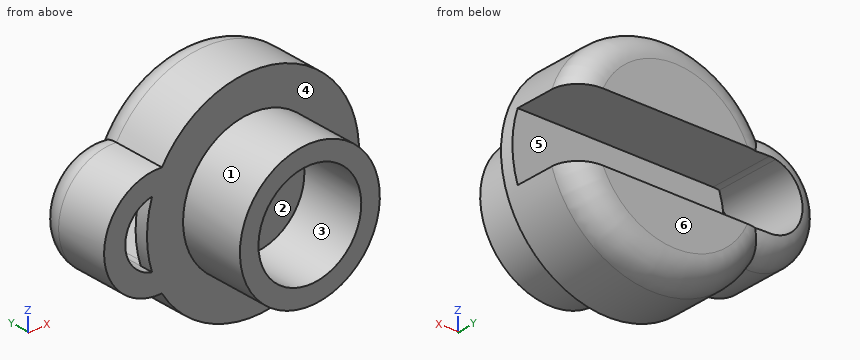
```python
from build123d import *

# Parameters (mm, degrees)
SKETCH1_R           = 3.3528
SKETCH1_R_2         = 2.4638
BOSS_EXTRUDE1_DEPTH = 3.175
SKETCH2_R           = 5.08
BOSS_EXTRUDE2_DEPTH = 3.81
BOSS_EXTRUDE3_START = -3.81
SKETCH3_R           = 5.08
SKETCH3_R_2         = 2.6035
SKETCH3_R_3         = 1.5875
BOSS_EXTRUDE3_DEPTH = 3.81
CUT_EXTRUDE1_START  = -3.175
CUT_EXTRUDE1_DEPTH  = 3.175
FILLET1_R           = 1.27


with BuildPart() as part:
    # Sketch1 → Boss-Extrude1 (new body)
    with BuildSketch(Plane(origin=(0, 0, 0), x_dir=(1, 0, 0), z_dir=(0, 1, 0))):
        with Locations(Location((0, 0, 0), (0, 0, 270))):
            Circle(SKETCH1_R)
        with Locations(Location((0, 0, 0), (0, 0, 270))):
            Circle(SKETCH1_R_2, mode=Mode.SUBTRACT)
    extrude(amount=BOSS_EXTRUDE1_DEPTH)

    # Sketch2 → Boss-Extrude2 (add)
    with BuildSketch(Plane(origin=(0, 3.175, 0), x_dir=(1, 0, 0), z_dir=(0, 1, 0))):
        with Locations(Location((0, 0, 0), (0, 0, 90))):
            Circle(SKETCH2_R)
    extrude(amount=BOSS_EXTRUDE2_DEPTH)

    # Sketch3 → Boss-Extrude3 (add)
    # profile 1 of 3: a face of its own
    with BuildSketch(Plane(origin=(0, 6.985, 0), x_dir=(1, 0, 0), z_dir=(0, 1, 0)).offset(BOSS_EXTRUDE3_START)):
        Circle(SKETCH3_R)
    # profile 2 of 3: a face of its own
    with BuildSketch(Plane(origin=(0, 6.985, 0), x_dir=(1, 0, 0), z_dir=(0, 1, 0)).offset(BOSS_EXTRUDE3_START)):
        with Locations((-4.533681302, 0)):
            Circle(SKETCH3_R_2)
        with Locations((-4.533681302, 0)):
            Circle(SKETCH3_R_3, mode=Mode.SUBTRACT)
    # profile 3 of 3: a face of its own
    with BuildSketch(Plane(origin=(0, 6.985, 0), x_dir=(1, 0, 0), z_dir=(0, 1, 0)).offset(BOSS_EXTRUDE3_START)):
        Circle(SKETCH3_R)
    extrude(amount=BOSS_EXTRUDE3_DEPTH)

    # Sketch4 → Cut-Extrude1 (cut)
    with BuildSketch(Plane(origin=(0, 6.985, 0), x_dir=(1, 0, 0), z_dir=(0, 1, 0)).offset(CUT_EXTRUDE1_START)):
        with BuildLine():
            ThreePointArc((-4.834979234, -1.558645504), (-4.685019521, -1.580269912), (-4.533681302, -1.5875))
            Line((-4.533681302, -1.5875), (4.825582219, -1.5875))
            ThreePointArc((4.825582219, -1.5875), (5.015992308, -0.803878824), (5.08, 0))
            ThreePointArc((5.08, 0), (5.015992308, 0.803878824), (4.825582219, 1.5875))
            Line((4.825582219, 1.5875), (-4.533681302, 1.5875))
            ThreePointArc((-4.533681302, 1.5875), (-4.685019521, 1.580269912), (-4.834979234, 1.558645504))
            ThreePointArc((-4.834979234, 1.558645504), (-5.08, 0), (-4.834979234, -1.558645504))
        make_face()
    extrude(amount=CUT_EXTRUDE1_DEPTH, mode=Mode.SUBTRACT)

    # Fillet1
    # the kernel refuses this fillet: 1.27 mm, written as the material it takes off along each edge
    with BuildSketch(Plane(origin=(-4.533681302, 6.985, 0), x_dir=(0.9598113025197432, 0, -0.2806461536443247), z_dir=(0.2806461536443247, 0, 0.9598113025197432))) as fillet1_piece_1_section:
        with BuildLine():
            CenterArc((2.6035 - FILLET1_R, -FILLET1_R), FILLET1_R, 0, 90)
            Line((2.6035, -FILLET1_R), (2.6035, 0))
            Line((2.6035, 0), (2.6035 - FILLET1_R, 0))
        make_face()
    fillet1_piece_1 = revolve(axis=Axis((-4.533681302, 6.985, 0), (0, 1, 0)), revolution_arc=327.402454095, mode=Mode.PRIVATE)
    fillet1_piece_1 = split(fillet1_piece_1, bisect_by=Plane(origin=(-4.533681302, 6.985, 1.5875), z_dir=(0, 0, -1)), keep=Keep.TOP, mode=Mode.PRIVATE)
    fillet1_piece_1 = split(fillet1_piece_1, bisect_by=Plane(origin=(-4.533681302, 6.985, -1.5875), z_dir=(0, 0, 1)), keep=Keep.TOP, mode=Mode.PRIVATE)
    add(fillet1_piece_1, mode=Mode.SUBTRACT)
    with BuildSketch(Plane(origin=(-4.533681302, 6.985, 0), x_dir=(0.9598113025197432, 0, -0.2806461536443247), z_dir=(0.2806461536443247, 0, 0.9598113025197432))) as fillet1_piece_2_section:
        with BuildLine():
            CenterArc((2.6035 - FILLET1_R, -FILLET1_R), FILLET1_R, 0, 90)
            Line((2.6035, -FILLET1_R), (2.6035, 0))
            Line((2.6035, 0), (2.6035 - FILLET1_R, 0))
        make_face()
    fillet1_piece_2 = revolve(axis=Axis((-4.533681302, 6.985, 0), (0, 1, 0)), revolution_arc=327.402454095, mode=Mode.PRIVATE)
    fillet1_piece_2 = fillet1_piece_2 - Plane(origin=(0, 6.985, 0), x_dir=(0, 0, -1), z_dir=(0, -1, 0)) * Cylinder(5.08, 11, mode=Mode.PRIVATE)
    add(fillet1_piece_2, mode=Mode.SUBTRACT)
    with BuildSketch(Plane(origin=(0, 6.985, 0), x_dir=(-0.9960699199988063, 0, 0.08857039275949603), z_dir=(0.08857039275949603, 0, 0.9960699199988063))) as fillet1_piece_3_section:
        with BuildLine():
            CenterArc((5.08 - FILLET1_R, FILLET1_R), FILLET1_R, 270, 90)
            Line((5.08 - FILLET1_R, 0), (5.08, 0))
            Line((5.08, 0), (5.08, FILLET1_R))
        make_face()
    fillet1_piece_3 = revolve(axis=Axis((0, 6.985, 0), (0, -1, 0)), revolution_arc=202.711774456, mode=Mode.PRIVATE)
    fillet1_piece_3 = fillet1_piece_3 - Plane(origin=(-4.533681302, 6.985, 0), x_dir=(1, 0, 0), z_dir=(0, -1, 0)) * Cylinder(2.6035, 21, mode=Mode.PRIVATE)
    add(fillet1_piece_3, mode=Mode.SUBTRACT)
    with BuildSketch(Plane(origin=(0, 6.985, 0), x_dir=(0.9530300689504536, 0, -0.30287569674091297), z_dir=(-0.30287569674091297, 0, -0.9530300689504536))) as fillet1_piece_4_section:
        with BuildLine():
            CenterArc((5.08 - FILLET1_R, FILLET1_R), FILLET1_R, 270, 90)
            Line((5.08 - FILLET1_R, 0), (5.08, 0))
            Line((5.08, 0), (5.08, FILLET1_R))
        make_face()
    fillet1_piece_4 = revolve(axis=Axis((0, 6.985, 0), (0, -1, 0)), revolution_arc=202.711774456, mode=Mode.PRIVATE)
    fillet1_piece_4 = fillet1_piece_4 - Plane(origin=(-4.533681302, 6.985, 0), x_dir=(1, 0, 0), z_dir=(0, -1, 0)) * Cylinder(2.6035, 21, mode=Mode.PRIVATE)
    add(fillet1_piece_4, mode=Mode.SUBTRACT)
    with BuildSketch(Plane(origin=(0, 6.985, 0), x_dir=(-0.9960699199988063, 0, 0.08857039275949603), z_dir=(0.08857039275949603, 0, 0.9960699199988063))) as fillet1_piece_5a_section:
        with BuildLine():
            CenterArc((5.08 - FILLET1_R, FILLET1_R), FILLET1_R, 270, 90)
            Line((5.08 - FILLET1_R, 0), (5.08, 0))
            Line((5.08, 0), (5.08, FILLET1_R))
        make_face()
    fillet1_piece_5a = revolve(axis=Axis((0, 6.985, 0), (0, -1, 0)), revolution_arc=202.711774456, mode=Mode.PRIVATE)
    fillet1_piece_5a = split(fillet1_piece_5a, bisect_by=Plane(origin=(0, 6.985, -1.5875), z_dir=(0, 0, -1)), keep=Keep.TOP, mode=Mode.PRIVATE)
    fillet1_piece_5a = fillet1_piece_5a & Plane(origin=(-4.533681302, 6.985, 0), x_dir=(1, 0, 0), z_dir=(0, -1, 0)) * Cylinder(2.6035, 21, mode=Mode.PRIVATE)
    with BuildSketch(Plane(origin=(-4.533681302, 6.985, 0), x_dir=(0.9598113025197432, 0, -0.2806461536443247), z_dir=(0.2806461536443247, 0, 0.9598113025197432))) as fillet1_piece_5b_section:
        with BuildLine():
            CenterArc((2.6035 - FILLET1_R, -FILLET1_R), FILLET1_R, 0, 90)
            Line((2.6035, -FILLET1_R), (2.6035, 0))
            Line((2.6035, 0), (2.6035 - FILLET1_R, 0))
        make_face()
    fillet1_piece_5b = revolve(axis=Axis((-4.533681302, 6.985, 0), (0, 1, 0)), revolution_arc=327.402454095, mode=Mode.PRIVATE)
    fillet1_piece_5b = fillet1_piece_5b & Plane(origin=(0, 6.985, 0), x_dir=(0, 0, -1), z_dir=(0, -1, 0)) * Cylinder(5.08, 11, mode=Mode.PRIVATE)
    fillet1_piece_5b = split(fillet1_piece_5b, bisect_by=Plane(origin=(-4.533681302, 6.985, -1.5875), z_dir=(0, 0, -1)), keep=Keep.TOP, mode=Mode.PRIVATE)
    fillet1_piece_5 = fillet1_piece_5a & fillet1_piece_5b
    add(fillet1_piece_5, mode=Mode.SUBTRACT)
    with BuildSketch(Plane(origin=(0, 6.985, 0), x_dir=(0.9530300689504536, 0, -0.30287569674091297), z_dir=(-0.30287569674091297, 0, -0.9530300689504536))) as fillet1_piece_6a_section:
        with BuildLine():
            CenterArc((5.08 - FILLET1_R, FILLET1_R), FILLET1_R, 270, 90)
            Line((5.08 - FILLET1_R, 0), (5.08, 0))
            Line((5.08, 0), (5.08, FILLET1_R))
        make_face()
    fillet1_piece_6a = revolve(axis=Axis((0, 6.985, 0), (0, -1, 0)), revolution_arc=202.711774456, mode=Mode.PRIVATE)
    fillet1_piece_6a = split(fillet1_piece_6a, bisect_by=Plane(origin=(0, 6.985, 1.5875), z_dir=(0, 0, 1)), keep=Keep.TOP, mode=Mode.PRIVATE)
    fillet1_piece_6a = fillet1_piece_6a & Plane(origin=(-4.533681302, 6.985, 0), x_dir=(1, 0, 0), z_dir=(0, -1, 0)) * Cylinder(2.6035, 21, mode=Mode.PRIVATE)
    with BuildSketch(Plane(origin=(-4.533681302, 6.985, 0), x_dir=(0.9598113025197432, 0, -0.2806461536443247), z_dir=(0.2806461536443247, 0, 0.9598113025197432))) as fillet1_piece_6b_section:
        with BuildLine():
            CenterArc((2.6035 - FILLET1_R, -FILLET1_R), FILLET1_R, 0, 90)
            Line((2.6035, -FILLET1_R), (2.6035, 0))
            Line((2.6035, 0), (2.6035 - FILLET1_R, 0))
        make_face()
    fillet1_piece_6b = revolve(axis=Axis((-4.533681302, 6.985, 0), (0, 1, 0)), revolution_arc=327.402454095, mode=Mode.PRIVATE)
    fillet1_piece_6b = fillet1_piece_6b & Plane(origin=(0, 6.985, 0), x_dir=(0, 0, -1), z_dir=(0, -1, 0)) * Cylinder(5.08, 11, mode=Mode.PRIVATE)
    fillet1_piece_6b = split(fillet1_piece_6b, bisect_by=Plane(origin=(-4.533681302, 6.985, 1.5875), z_dir=(0, 0, 1)), keep=Keep.TOP, mode=Mode.PRIVATE)
    fillet1_piece_6 = fillet1_piece_6a & fillet1_piece_6b
    add(fillet1_piece_6, mode=Mode.SUBTRACT)


solid = part.part
```
Check sheet for the modelled part. Datum: model origin and axes. Units: mm. Face numbers are marked on the shaded views. A direction names the side the tool comes from. Coordinates: 2 decimals unless noted, no trailing zeros. Order: outer loops, then holes, each group sorted by start corner. A loop starts at its lowest first (then second) coordinate and runs counter-clockwise, first axis right, second up. Notation, with made-up numbers: M 43.25,9 L 64.25,9 A23 ccw 64.25,40 Z; hole C 35.25,-29 d10. An arc over 180 degrees is marked long. Write each question's results on one line, items separated by ' | '. Start each with the question number.
1. Cross-section at C-C on y = 2.75. Record the cut outline in (x, z).
2. Cross-section at A-A on z = 0. Record the cut outline in (x, y) (3 decimals), and give its area (3 significant figures).
3. Material ranges on probe 1 along X at (y, z) = (2.25, 0); probe 2 along Y at (x, z) = (3.75, 1) (3 decimals); probe 3 along Y at (x, z) = (2.75, 0.5), recorded low to high.
4. Mould release check, pull along X, two halves, no side actions. Record for the marked faces 1, 2, 3 and 4: +X half, -X half, draft (parallel to the pull), parting line (faces both ways), or undercut.
5. Go/stop test with flat-tipped pins: P1, Ø4, axis at x = -5, z = -3, coming from the -Y side (3 decimals); P2, Ø1, axis at x = 1, y = 5.5, coming from the -Z side; P3, Ø1.5, axis at x = 2, y = 3, coming from the -Z side. Record where each tip stops, or that it passes through.
6. Access from +Z, -Z, +X, -X, +Y, -Y to the whole of each face (thin tool, end or side, straight path). Record for the marked faces 5 and 6.
7. Cross-section at B-B on x = 0. Record the cut outline in (y, z) (1 decimal), and give its area (3 significant figures).
8. Cross-section at D-D on y = 6. Record the cut outline in (x, z) (1 decimal), and give its area (3 significant figures).
Checks:
1) outline: C 0,0 d6.71; hole C 0,0 d4.93
2) outline: M -7.137,3.175 L -6.121,3.175 L -6.121,6.959 A1.27 ccw -7.137,5.715 Z; M -5.08,3.175 L -3.353,3.175 L -3.353,0 L -2.464,0 L -2.464,3.175 L 2.464,3.175 L 2.464,0 L 3.353,0 L 3.353,3.175 L 5.08,3.175 L 5.08,3.81 L -5.08,3.81 Z | area: 15.6 mm²
3) probe 1: x = -3.35 to -2.46, 2.46 to 3.35 | probe 2: y = 3.175 to 3.81 | probe 3: y = 0 to 3.81
4) face 1: parting line | face 2: undercut | face 3: undercut | face 4: draft
5) P1: stops at y = 3.175 | P2: stops at z = -5.06 | P3: stops at z = -4.92
6) face 5: +X, +Y | face 6: +Z, -Z, +X, -X, +Y
7) outline: M 0,-3.4 L 3.2,-3.4 L 3.2,-5.1 L 5.7,-5.1 A1.3 ccw 7,-3.8 L 7,-1.6 L 3.8,-1.6 L 3.8,1.6 L 7,1.6 L 7,3.8 A1.3 ccw 5.7,5.1 L 3.2,5.1 L 3.2,3.4 L 0,3.4 L 0,2.5 L 3.2,2.5 L 3.2,-2.5 L 0,-2.5 Z | area: 33.6 mm²
8) outline: M -4.5,-1.6 A1.6 cw -4.5,1.6 L 4.8,1.6 A5 ccw -4.3,2.6 A2.6 ccw long -4.3,-2.6 A5 ccw 4.8,-1.6 Z | area: 54.8 mm²
